```python
from build123d import *

# Parameters (mm, degrees)
SKETCH1_R           = 1
BOSS_EXTRUDE1_DEPTH = 10
SKETCH2_R           = 2.5
CUT_EXTRUDE1_DEPTH  = 11


with BuildPart() as part:
    # Sketch1 → Boss-Extrude1 (new body)
    with BuildSketch(Plane.XY):
        with BuildLine():
            Line((5, 0), (145, 0))
            ThreePointArc((145, 0), (148.535533906, 1.464466094), (150, 5))
            Line((150, 5), (150, 25))
            ThreePointArc((150, 25), (148.535533906, 28.535533906), (145, 30))
            Line((145, 30), (5, 30))
            ThreePointArc((5, 30), (1.464466094, 28.535533906), (0, 25))
            Line((0, 25), (0, 5))
            ThreePointArc((0, 5), (1.464466094, 1.464466094), (5, 0))
        make_face()
        with Locations((25, 15)):
            Circle(SKETCH1_R, mode=Mode.SUBTRACT)
        with Locations((125, 15)):
            Circle(SKETCH1_R, mode=Mode.SUBTRACT)
    extrude(amount=BOSS_EXTRUDE1_DEPTH)

    # Sketch2 → Cut-Extrude1 (cut, through all)
    with BuildSketch(Plane.XY.offset(10)):
        with Locations((15, 25)):
            Circle(SKETCH2_R)
        with Locations((15, 5)):
            Circle(SKETCH2_R)
        with Locations((135, 25)):
            Circle(SKETCH2_R)
        with Locations((135, 5)):
            Circle(SKETCH2_R)
    extrude(amount=-CUT_EXTRUDE1_DEPTH, mode=Mode.SUBTRACT)


solid = part.part
```
Model file for the job. Use its own axes, mm. Coordinates: 2 decimals unless noted, no trailing zeros. Write each loop counter-clockwise with the first axis right and the second up, starting at its lowest first coordinate (ties: lowest second). Pieces come first, ordered by that corner, then holes. Notation, with made-up numbers: (-8.5, 36) - (42.5, 36) arc R27 cw to (42.5, 57) - close; hole circle Ø3 at (89.5, 70). An arc over 180 degrees is marked (long way). Use a Markdown table: item, result. Add a question column.
Item 1: Drill centre lines: line 1 along Y through (x, z) = (135, 8.25); line 2 along Y through (x, z) = (125, 5.25); line 3 along X through (y, z) = (15.75, 4.75). Where is each one in solid material? Low to high.
Item 2: Two-plate mould, pull along X, no slides. Class faces 1 (the face through (74, 15, 10)), 2 (the face through (137.385, 25.751, 5.07)), 3 (the face through (0, 15, 5)): pulls with the +X half, pulls with the -X half, needs draft (parallel to the pull), parting line crosses it, or undercut.
Item 3: Band-saw the part on B-B, the plane z = 4.75. Write the cut outline in (x, y), and give its area (3 significant figures).
Item 4: Band-saw the part on A-A, the plane x = 135. Write the cut outline in (y, z).
Item 5: Drop a flat-ended pin along its axis: pin 1 (1.6 mm diameter, centred on x = 125, y = 15, fed in from -Z). Give the stop position or say it passes through.
A:
| question | item | result |
|---|---|---|
| 1 | line 1 | y = 0 to 2.5, 7.5 to 22.5, 27.5 to 30 |
| 1 | line 2 | y = 0 to 14, 16 to 30 |
| 1 | line 3 | x = 0 to 24.34, 25.66 to 124.34, 125.66 to 150 |
| 2 | face 1 | needs draft |
| 2 | face 2 | undercut |
| 2 | face 3 | pulls with the -X half |
| 3 | outline | (0, 5) arc R5 ccw to (5, 0) - (145, 0) arc R5 ccw to (150, 5) - (150, 25) arc R5 ccw to (145, 30) - (5, 30) arc R5 ccw to (0, 25) - close; hole circle Ø5 at (15, 5); hole circle Ø5 at (15, 25); hole circle Ø2 at (25, 15); hole circle Ø2 at (125, 15); hole circle Ø5 at (135, 5); hole circle Ø5 at (135, 25) |
| 3 | area | 4,390 mm² |
| 4 | outline | (0, 0) - (2.5, 0) - (2.5, 10) - (0, 10) - close; (7.5, 0) - (22.5, 0) - (22.5, 10) - (7.5, 10) - close; (27.5, 0) - (30, 0) - (30, 10) - (27.5, 10) - close |
| 5 | pin 1 | passes through |
